For this review, use the dimensioned drawing (mm, ordinates from the lowest corner) and the shaded views. Give positions to 0.01 mm unless a question says otherwise; leave off trailing zeros. Loops run counter-clockwise (first coordinate to the right, second up) from the corner with the lowest first, then second, coordinate; pieces in that order, holes last. Notation, with made-up numbers: M 60,-31 L 65,-31 A16 ccw 65,-7 Z; hole C -26,19 d2. An arc over 180 degrees is marked long. Use a Markdown table: item, result. Add a question column.
(1) Add section A-A, the plane x = 293. Give the boundary of the cut face in (y, z), then the cut area to 3 significant figures.
(2) Insertion check: pin 1 Ø3.5 at (x, z) = (128, 133) entering from -Y; pin 2 Ø0.9 at (x, y) = (287, 1.5) entering from -Z. Each pin has a flat end and moves straight along its axis. Give the tip position at first contact, or say it passes through.
(3) For probe 1 along X at (y, z) = (0.25, 43); probe 2 along Z at (x, y) = (21, 1.4); probe 3 along X at (y, z) = (1.8, 133), list the stretches that pass through material, from the lowest coordinate up.
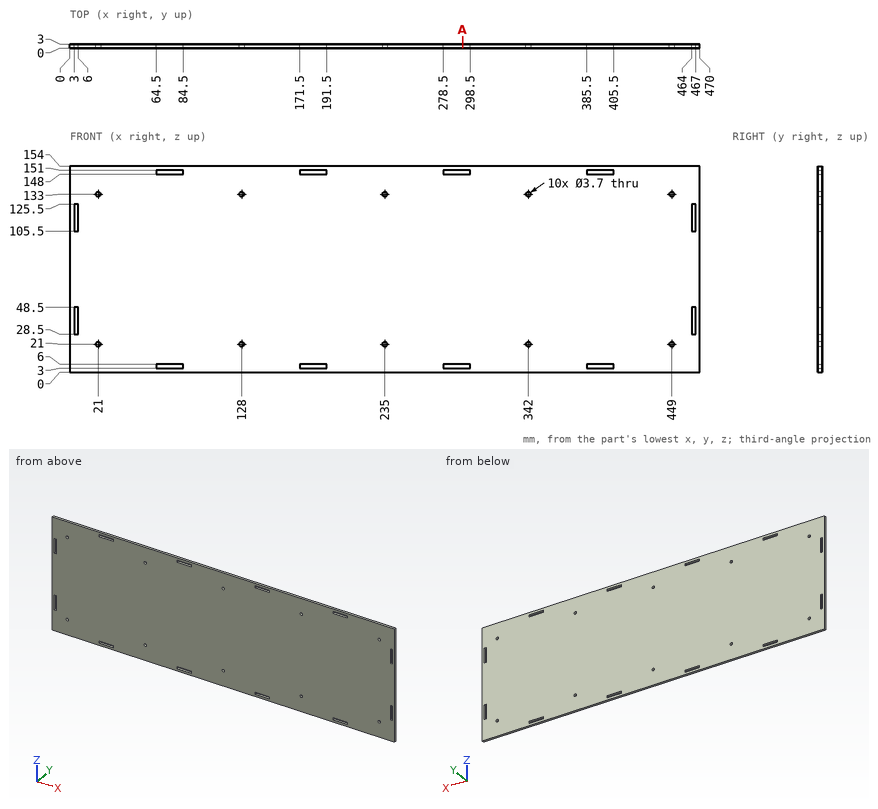
Established:
| question | item | result |
|---|---|---|
| 1 | outline | M 0,0 L 3,0 L 3,3 L 0,3 Z; M 0,6 L 3,6 L 3,148 L 0,148 Z; M 0,151 L 3,151 L 3,154 L 0,154 Z |
| 1 | area | 444 mm^2 |
| 2 | pin 1 | through |
| 2 | pin 2 | z = 0 |
| 3 | probe 1 | 0 to 3, 6 to 464, 467 to 470 |
| 3 | probe 2 | 0 to 19.15, 22.85 to 131.15, 134.85 to 154 |
| 3 | probe 3 | 0 to 19.15, 22.85 to 126.15, 129.85 to 233.15, 236.85 to 340.15, 343.85 to 447.15, 450.85 to 470 |
